Source: CAD feature listing. Evaluate the final solid. Frame: model axes, mm. A direction names the side the tool comes from. Give positions to 0.01 mm unless a question says otherwise; leave off trailing zeros. Loops run counter-clockwise (first coordinate to the right, second up) from the corner with the lowest first, then second, coordinate; pieces in that order, holes last. Notation, with made-up numbers: (26, 68) - (59, 68) arc R13 cw to (59, 90) - close; hole circle Ø9 at (-25, -5). An arc over 180 degrees is marked (long way). Write each question's results on one line, items separated by ' | '. Start each with the question number.
(1) Pull-direction query (X, two-part tool) for faces 1 (the flat face through (80, 53.594, 54)), 2 (the flat face through (76.636, 44, 69)), 3 (the cylindrical face through (-30.55, 0.31, 46.86)); classes: pulls with the +X half, pulls with the -X half, needs draft (parallel to the pull), parting line crosses it, or undercut.
(2) Cut plane C-C on y = -16. Return the cut outline in (x, z), then the cut area to 3 significant figures.
(3) Contact query for flat-ended pins moving along their axis: pin 1 (1.5 mm diameter, centred on x = -52.5, y = 33.5, fed in from +Z); pin 2 (4 mm diameter, centred on y = -33, z = 32, fed in from -X); pin 3 (6.5 mm diameter, centred on y = -39, z = 75.5, fed in from -X). Output: stop coordinate, or through.
(4) Cut plane A-A on x = 40.5. Return the cut outline in (y, z), then the cut area to 3 significant figures.
(5) Reachability of faces 4 (the flat face through (30, 54.864, 13)), 5 (the flat face through (80, -53.594, 54)), 6 (the flat face through (-27, 22.098, 43)) from +Z, -Z, +X, -X, +Y, -Y: full face, straight path, thin tool, end or side. Return the list, or none.
(6) Material intervals for line 1 along Y through (x, z) = (96, 57); line 2 along Z through (x, y) = (-52, -42.5); line 3 along Z through (x, y) = (51.5, 19), sorted ascending. Write a range as [from, to].
(7) Cut plane B-B on z = 60. Return the cut outline in (x, y).
(8) Cut plane D-D on z = 30. Return the cut outline in (x, y).
from build123d import *

# Parameters (mm, degrees)
F1_DEPTH    = 54.864
F0_R        = 15.7777597409
F2_DEPTH    = 22.098
F3_DEPTH    = 53.594
F4_T1_DEPTH = 332.0051224214
F5_DEPTH    = 131.826
F6_W        = 67.7949339151
F6_H        = 61.7567202186
F7_DEPTH    = 41.148


# Not quite as in the source:
# - a fillet or chamfer that OpenCascade refuses, or shapes differently, is made with other operations: its cross-section is extruded or revolved along the edge and cut away or added


with BuildPart() as f1:
    # F0 (on Front) → F1 (new body, symmetric)
    with BuildSketch(Plane.XZ):
        Polygon((-107.4633456931, 25.4), (-107.4633456931, 0), (107.6379133128, 0), (107.6379133128, 25.4), (11.4811650322, 25.4), (-65.0678679326, 25.4), align=None)
    extrude(amount=F1_DEPTH, both=True)

    # F0 (on Front) → F2 (join, symmetric)
    with BuildSketch(Plane.XZ):
        with BuildLine():
            Line((-46.6904140055, 63.9219704105), (-65.0678679326, 25.4))
            Line((-65.0678679326, 25.4), (11.4811650322, 25.4))
            Line((11.4811650322, 25.4), (11.4811650322, 39.0391899168))
            Line((11.4811650322, 39.0391899168), (11.4811650322, 53.899857424))
            ThreePointArc((11.4811650322, 53.899857424), (-7.5633921192, 84.1691084188), (-41.8619237654, 74.0432287141))
            Line((-41.8619237654, 74.0432287141), (-46.6904140055, 63.9219704105))
        make_face()
        with Locations((-18.0268805863, 56.4600032051)):
            Circle(F0_R, mode=Mode.SUBTRACT)
    extrude(amount=F2_DEPTH, both=True)

    # F0 (on Front) → F3 (join, symmetric)
    with BuildSketch(Plane.XZ):
        Polygon((11.4811650322, 25.4), (107.6379133128, 25.4), (107.6379133128, 98.0671415215), (76.6363167746, 98.0671415215), (76.6363167746, 39.0391899168), (11.4811650322, 39.0391899168), align=None)
    extrude(amount=F3_DEPTH, both=True)

    # F4: fillet of radius 61.3210244843 on 2 edges, made by hand

    # F4_s2 → F4_t1 (cut)
    with BuildSketch(Plane.XY.offset(-153.3025612107)):
        with BuildLine():
            ThreePointArc((-107.4633456931, -6.4570244843), (-89.502833451, 36.9034877579), (-46.1423212089, 54.864))
            Line((-46.1423212089, 54.864), (-107.4633456931, 54.864))
            Line((-107.4633456931, 54.864), (-107.4633456931, -6.4570244843))
        make_face()
        with BuildLine():
            ThreePointArc((-107.4633456931, 6.4570244843), (-89.502833451, -36.9034877579), (-46.1423212089, -54.864))
            Line((-46.1423212089, -54.864), (-107.4633456931, -54.864))
            Line((-107.4633456931, -54.864), (-107.4633456931, 6.4570244843))
        make_face()
    extrude(amount=F4_T1_DEPTH, mode=Mode.SUBTRACT)

    # F0 (on Front) → F5 (cut)
    with BuildSketch(Plane.XZ):
        with Locations((-18.0268805863, 56.4600032051)):
            Circle(F0_R)
    extrude(amount=-F5_DEPTH, mode=Mode.SUBTRACT)

    # F6 (on face) → F7 (cut)
    with BuildSketch(Plane.YZ.offset(107.6379133128)):
        with Locations((1.151856035, 67.1887814122)):
            Rectangle(F6_W, F6_H)
    extrude(amount=-F7_DEPTH, mode=Mode.SUBTRACT)


solid = f1.part
Ans:
1) face 1: needs draft | face 2: pulls with the -X half | face 3: undercut
2) outline: (-103.2, 0) - (107.64, 0) - (107.64, 36.31) - (66.49, 36.31) - (66.49, 39.04) - (11.48, 39.04) - (11.48, 53.9) arc R29.62 ccw to (-41.86, 74.04) - (-65.07, 25.4) - (-103.2, 25.4) - close; hole circle Ø31.56 at (-18.03, 56.46) | area: 9,300 mm^2
3) pin 1: z = 25.4 | pin 2: x = 11.48 | pin 3: x = 76.64
4) outline: (-54.86, 0) - (54.86, 0) - (54.86, 25.4) - (53.59, 25.4) - (53.59, 39.04) - (-53.59, 39.04) - (-53.59, 25.4) - (-54.86, 25.4) - close | area: 4,250 mm^2
5) face 4: +Z, -Z, +X, -X, +Y | face 5: +Z, +X, -X, -Y | face 6: +Z, -X, +Y
6) line 1: [-53.59, -32.75], [35.05, 53.59] | line 2: [0, 25.4] | line 3: [0, 39.04]
7) outline: (-48.56, -22.1) - (-33.4, -22.1) - (-33.4, 22.1) - (-48.56, 22.1) - close; (-2.65, -22.1) - (11.38, -22.1) - (11.38, 22.1) - (-2.65, 22.1) - close; (76.64, -53.59) - (107.64, -53.59) - (107.64, -32.75) - (76.64, -32.75) - close; (76.64, 35.05) - (107.64, 35.05) - (107.64, 53.59) - (76.64, 53.59) - close
8) outline: (-62.87, -22.1) - (11.48, -22.1) - (11.48, -53.59) - (107.64, -53.59) - (107.64, 53.59) - (11.48, 53.59) - (11.48, 22.1) - (-62.87, 22.1) - close
